```python
from build123d import *

# Parameters (mm, degrees)
F1_DEPTH = 25.4


with BuildPart() as f1:
    # F0 (on Front) → F1 (new body)
    with BuildSketch(Plane.XZ):
        with BuildLine():
            Line((-101.6, 0), (-76.2, 0))
            Line((-76.2, 0), (-76.2, 3.175))
            Line((-76.2, 3.175), (-83.856648, 3.175))
            ThreePointArc((-83.856648, 3.175), (-76.460894, 4.14867), (-69.569148, 7.003324))
            Line((-69.569148, 7.003324), (-49.493352, 18.594091))
            ThreePointArc((-49.493352, 18.594091), (-37.241359, 23.669032), (-24.093352, 25.4))
            Line((-24.093352, 25.4), (0, 25.4))
            Line((0, 25.4), (0, 28.575))
            Line((0, 28.575), (-23.242613, 28.575))
            ThreePointArc((-23.242613, 28.575), (-37.212371, 26.735846), (-50.230113, 21.343721))
            Line((-50.230113, 21.343721), (-70.305909, 9.752955))
            ThreePointArc((-70.305909, 9.752955), (-76.431906, 7.215484), (-83.005909, 6.35))
            Line((-83.005909, 6.35), (-93.82287, 6.35))
            ThreePointArc((-93.82287, 6.35), (-96.222944, 6.821042), (-98.266944, 8.164286))
            ThreePointArc((-98.266944, 8.164286), (-106.009218, 6.562556), (-101.6, 0))
        make_face()
        with BuildLine():
            ThreePointArc((-100.488981, 5.896429), (-97.422982, 3.881564), (-93.82287, 3.175))
            Line((-93.82287, 3.175), (-101.6, 3.175))
            ThreePointArc((-101.6, 3.175), (-103.069739, 5.362519), (-100.488981, 5.896429))
        make_face(mode=Mode.SUBTRACT)
        with BuildLine():
            Line((0, 28.575), (0, 25.4))
            Line((0, 25.4), (24.093352, 25.4))
            ThreePointArc((24.093352, 25.4), (37.241359, 23.669032), (49.493352, 18.594091))
            Line((49.493352, 18.594091), (69.569148, 7.003324))
            ThreePointArc((69.569148, 7.003324), (76.460894, 4.14867), (83.856648, 3.175))
            Line((83.856648, 3.175), (76.2, 3.175))
            Line((76.2, 3.175), (76.2, 0))
            Line((76.2, 0), (101.6, 0))
            ThreePointArc((101.6, 0), (106.009218, 6.562556), (98.266944, 8.164286))
            ThreePointArc((98.266944, 8.164286), (96.222944, 6.821042), (93.82287, 6.35))
            Line((93.82287, 6.35), (83.005909, 6.35))
            ThreePointArc((83.005909, 6.35), (76.431906, 7.215484), (70.305909, 9.752955))
            Line((70.305909, 9.752955), (50.230113, 21.343721))
            ThreePointArc((50.230113, 21.343721), (37.212371, 26.735846), (23.242613, 28.575))
            Line((23.242613, 28.575), (0, 28.575))
        make_face()
        with BuildLine():
            Line((101.6, 3.175), (93.82287, 3.175))
            ThreePointArc((93.82287, 3.175), (97.422982, 3.881564), (100.488981, 5.896429))
            ThreePointArc((100.488981, 5.896429), (103.069739, 5.362519), (101.6, 3.175))
        make_face(mode=Mode.SUBTRACT)
    extrude(amount=F1_DEPTH)


solid = f1.part
```
Work out the finished part from the listing and answer in its coordinate system (mm). A direction names the side the tool comes from. Coordinates: 2 decimals unless noted, no trailing zeros. Loops run counter-clockwise (first coordinate to the right, second up) from the corner with the lowest first, then second, coordinate; pieces in that order, holes last. Notation, with made-up numbers: M 75,86.25 L 106,86.25 A25 ccw 106,102.25 Z; hole C 61.25,50.5 d2. An arc over 180 degrees is marked long. Use CSV: the item, a comma, the result in double quotes. Start each with the question number.
(1) Consider line 1 (Z direction, x = -101.6, y = -12.5) (3 decimals); line 2 (X direction, y = -2.75, z = 5.5); line 3 (X direction, y = -13.5, z = 17.5). Determine where each line is inside the solid, lowest interval first.
(2) Given pin 1 Ø8.5 at (x, y) = (90.5, -14) entering from +Z; pin 2 Ø4 at (x, y) = (-97.5, -15) entering from +Z; pin 3 Ø4 at (y, z) = (-4, 21) entering from -X, each flat-ended and moving along its own axis, determine where each tip first touches the part or whether it passes through.
(3) Find section A-A, the plane y = -11. State how many separate pieces and enclosed holes the cut face has, then the cut area to 3 significant figures.
(4) Find section B-B, the plane x = 87.5. Give the vertices of the cut face in (y, z).
(5) For faces 1 (the face through (-59.7, -12.5, 12.7)), 2 (the face through (-76.34, -12.52, 7.24)), 3 (the face through (106.057, -12.522, 6.441)), determine the directions among +Z, -Z, +X, -X, +Y, -Y from which every point of the face is accessible in a straight line to the end or side of a thin tool.
(6) Find section C-C, the plane x = -10. Give the vertices of the cut face in (y, z) (3 decimals), then the cut area to 3 significant figures.
Recorded:
1,line 1,"z = 0 to 3.175, 6.35 to 9.525"
1,line 2,"x = -106.31 to -103.01, -100.06 to -72.57, 72.57 to 100.06, 103.01 to 106.31"
1,line 3,"x = -56.89 to -51.39, 51.39 to 56.89"
2,pin 1,"stops at z = 6.42"
2,pin 2,"stops at z = 9.04"
2,pin 3,"stops at x = -54.29"
3,separate pieces,"1"
3,enclosed holes,"2"
3,area,"869 mm^2"
4,outline,"M -25.4,0 L 0,0 L 0,6.35 L -25.4,6.35 Z"
5,face 1,"-Z, +Y, -Y"
5,face 2,"+Z, +Y, -Y"
5,face 3,"+Y, -Y"
6,outline,"M -25.4,25.4 L 0,25.4 L 0,28.575 L -25.4,28.575 Z"
6,area,"80.6 mm^2"
